Could you check a few things on this model? Use its own coordinates, in mm. A direction names the side the tool comes from. Coordinates: 2 decimals unless noted, no trailing zeros. Order: outer loops, then holes, each group sorted by start corner. A loop starts at its lowest first (then second) coordinate and runs counter-clockwise, first axis right, second up. Notation, with made-up numbers: (9.25, -9) - (59.25, -9) arc R22 cw to (59.25, 23) - close; hole circle Ø5 at (30.25, 58.5). An arc over 180 degrees is marked (long way). Answer as a JSON object with one key per item and string values. Group by question number.
(1) Imagine slicing it at B-B, the plane x = 7. Give the number of separate pieces and of enclosed holes in the cut face, and give its area (3 significant figures).
(2) Which directions (+Z, -Z, +X, -X, +Y, -Y) give clear straight access to the entire face, cutting with the end or side of a thin tool? Please do faces 4 (the flat face through (-0.5, 5, 0)), 5 (the flat face through (6.86, 35.49, 14.88)), 6 (the flat face through (16, 35, -1.5)), 7 (the flat face through (-16, 35, 1.5)).
(3) Please list where these lines run through material, in increasing order: probe 1 along Z at (x, y) = (5.5, 21.5); probe 2 along Z at (x, y) = (17.5, 36.5); probe 3 along X at (y, z) = (55, 16.5).
(4) Imagine slicing it at D-D, the plane y = 21.5. Write out the boundary of the cut face in (x, z).
(5) Imagine slicing it at C-C, the plane x = 28. Write out the boundary of the cut face in (y, z), and give its area (3 significant figures).
(6) We'd pull the mould along X, two halves only. Please class faces 1 (the cylindrical face through (-17.478, 34.297, -30.315)), 2 (the cylindrical face through (1.5, 4.9, 0)), 3 (the flat face through (-1, 0, 0)): pulls with the +X half, pulls with the -X half, needs draft (parallel to the pull), parting line crosses it, or undercut.
(7) Will these pins go through, and if not, where does the flat tip stop? P1, Ø6, axis at y = 50.5, z = 9.5, coming from the -X side; P2, Ø1.5, axis at y = 35.5, z = -10, coming from the -X side; P3, Ø2, axis at x = -11, z = -22.5, coming from the +Y side.
(8) Imagine slicing it at A-A, the plane y = 42.5. Write out the boundary of the cut face in (x, z), and give its area (3 significant figures).
from build123d import *

# Parameters (mm, degrees)
SKETCH2_R           = 5
BOSS_EXTRUDE1_DEPTH = 80
BOSS_EXTRUDE2_DEPTH = 1.5
CIRPATTERN1_COUNT   = 6
CUT_EXTRUDE1_DEPTH  = 10


with BuildPart() as part:
    # Sketch2 → Boss-Extrude1 (new body)
    with BuildSketch(Plane(origin=(0, 0, 0), x_dir=(1, 0, 0), z_dir=(0, 1, 0))):
        with Locations(Location((0, 0, 0), (0, 0, 270))):
            Circle(SKETCH2_R)
    extrude(amount=BOSS_EXTRUDE1_DEPTH)

    # Sketch3 → Boss-Extrude2 (add, symmetric)
    with BuildSketch(Plane.XY):
        with BuildLine():
            Line((0, 70), (0, 0))
            ThreePointArc((0, 0), (35, 35), (0, 70))
        make_face()
    boss_extrude2 = extrude(amount=BOSS_EXTRUDE2_DEPTH, both=True)

    # CirPattern1: Boss-Extrude2 ×6 about axis
    cirpattern1_axis = Axis((0, 0, 0), (0, 1, 0))
    for i in range(1, CIRPATTERN1_COUNT):
        add(boss_extrude2.rotate(cirpattern1_axis, i * 360 / CIRPATTERN1_COUNT))

    # Sketch4 → Cut-Extrude1 (cut)
    with BuildSketch(Plane.XZ):
        with BuildLine():
            Line((-0.5, 1.414213562), (-0.5, -1.414213562))
            ThreePointArc((-0.5, -1.414213562), (1.5, 0), (-0.5, 1.414213562))
        make_face()
    extrude(amount=-CUT_EXTRUDE1_DEPTH, mode=Mode.SUBTRACT)


solid = part.part
Result set:
{
 "1": {"separate pieces": "3", "enclosed holes": "0", "area": "975 mm^2"},
 "2": {"face 4": "-Y", "face 5": "+Z, +Y, -Y", "face 6": "+X, +Y, -Y", "face 7": "-X, +Y, -Y"},
 "3": {"probe 1": "z = -12.53 to -6.53, -1.5 to 1.5, 6.53 to 12.53", "probe 2": "z = -30.27 to -27.31, -1.5 to 1.5, 27.31 to 30.27", "probe 3": "x = -11.26 to -7.79, 7.79 to 11.26"},
 "4": {"outline": "(-32.29, -1.5) - (-4.77, -1.5) arc R5 ccw to (-3.68, -3.38) - (-17.44, -27.22) - (-14.85, -28.72) - (-1.09, -4.88) arc R5 ccw to (1.09, -4.88) - (14.85, -28.72) - (17.44, -27.22) - (3.68, -3.38) arc R5 ccw to (4.77, -1.5) - (32.29, -1.5) - (32.29, 1.5) - (4.77, 1.5) arc R5 ccw to (3.68, 3.38) - (17.44, 27.22) - (14.85, 28.72) - (1.09, 4.88) arc R5 ccw to (-1.09, 4.88) - (-14.85, 28.72) - (-17.44, 27.22) - (-3.68, 3.38) arc R5 ccw to (-4.77, 1.5) - (-32.29, 1.5) - close"},
 "5": {"outline": "(14, -1.5) - (56, -1.5) - (56, 1.5) - (14, 1.5) - close", "area": "126 mm^2"},
 "6": {"face 1": "pulls with the -X half", "face 2": "undercut", "face 3": "needs draft"},
 "7": {"P1": "stops at x = -8.95", "P2": "stops at x = -7.94", "P3": "stops at y = 60.47"},
 "8": {"outline": "(-34.19, -1.5) - (-4.77, -1.5) arc R5 ccw to (-3.68, -3.38) - (-18.39, -28.86) - (-15.79, -30.36) - (-1.09, -4.88) arc R5 ccw to (1.09, -4.88) - (15.79, -30.36) - (18.39, -28.86) - (3.68, -3.38) arc R5 ccw to (4.77, -1.5) - (34.19, -1.5) - (34.19, 1.5) - (4.77, 1.5) arc R5 ccw to (3.68, 3.38) - (18.39, 28.86) - (15.79, 30.36) - (1.09, 4.88) arc R5 ccw to (-1.09, 4.88) - (-15.79, 30.36) - (-18.39, 28.86) - (-3.68, 3.38) arc R5 ccw to (-4.77, 1.5) - (-34.19, 1.5) - close", "area": "605 mm^2"}
}
